```python
from build123d import *

# Parameters (mm, degrees)
SKETCH1_W               = 120.517011816
SKETCH1_H               = 193.423301163
BOSS_EXTRUDE1_DEPTH     = 75
SKETCH1_3_W             = 118.517011816
SKETCH1_3_H             = 191.423301163
CUT_EXTRUDE1_DEPTH      = 70
BOSS_EXTRUDE2_DEPTH     = 1
CUT_EXTRUDE4_DEPTH      = 137.495747048
CUT_EXTRUDE4_DEPTH_BACK = 137.495747048
CUT_EXTRUDE6_DEPTH      = 10
CUT_EXTRUDE3_DEPTH      = 10


with BuildPart() as part:
    # Sketch1 → Boss-Extrude1 (new body)
    with BuildSketch(Plane.XY):
        with Locations((0.026299542, -0.057021664)):
            Rectangle(SKETCH1_W, SKETCH1_H)
    extrude(amount=BOSS_EXTRUDE1_DEPTH)

    # Sketch1_3 → Cut-Extrude1 (cut)
    with BuildSketch(Plane.XY):
        with Locations((0.026299542, -0.057021664)):
            Rectangle(SKETCH1_3_W, SKETCH1_3_H)
    extrude(amount=CUT_EXTRUDE1_DEPTH, mode=Mode.SUBTRACT)

    # Sketch2 → Boss-Extrude2 (add)
    with BuildSketch(Plane(origin=(0, 96.654628917, 0), x_dir=(1, 0, 0), z_dir=(0, 1, 0))):
        with BuildLine():
            Line((-5.120692539, 0), (4.878786885, 0))
            ThreePointArc((4.878786885, 0), (-0.120952827, 5.051017752), (-5.120692539, 0))
        make_face()
    extrude(amount=-BOSS_EXTRUDE2_DEPTH)

    # Sketch4_2 → Cut-Extrude4 (cut, two sides: drawn at the far end of the back side and taken through both)
    with BuildSketch(Plane(origin=(0, 0, 70), x_dir=(-1, 0, 0), z_dir=(0, 0, -1)).offset(-CUT_EXTRUDE4_DEPTH_BACK)):
        with BuildLine():
            Line((-16.236705508, 8.803847843), (-16.236705508, 26.966349614))
            add(Edge.make_bspline(
                [(10.654600955, 26.966349614), (10.654600955, 37.042694246), (-2.791052277, 37.042694246), (-16.236705508, 37.042694246), (-16.236705508, 26.966349614)],
                knots=[3.141592654, 3.141592654, 3.141592654, 4.71238898, 4.71238898, 6.283185307, 6.283185307, 6.283185307], degree=2, weights=[1, 0.707106781, 1, 0.707106781, 1]))
            Line((10.654600955, 26.966349614), (10.654600955, 8.803847843))
            add(Edge.make_bspline(
                [(-16.236705508, 8.803847843), (-16.236705508, 0.726850718), (-2.791052277, 0.726850718), (10.654600955, 0.726850718), (10.654600955, 8.803847843)],
                knots=[0, 0, 0, 1.570796327, 1.570796327, 3.141592654, 3.141592654, 3.141592654], degree=2, weights=[1, 0.707106781, 1, 0.707106781, 1]))
        make_face()
    extrude(amount=CUT_EXTRUDE4_DEPTH + CUT_EXTRUDE4_DEPTH_BACK, mode=Mode.SUBTRACT)

    # Sketch6 → Cut-Extrude6 (cut, symmetric)
    with BuildSketch(Plane(origin=(0, 96.654628917, 0), x_dir=(1, 0, 0), z_dir=(0, 1, 0))):
        with BuildLine():
            add(Edge.make_bspline(
                [(14.607126744, -59.625274066), (14.607126744, -59.996423236), (14.655753616, -60.360654617), (14.797863596, -60.897161426), (14.856849596, -61.074344505), (14.9984446, -61.42534999), (15.081484622, -61.59993657), (15.36467279, -62.113067792), (15.595340891, -62.436179632), (16.002179988, -62.893279801), (16.148006268, -63.041018505), (16.460654262, -63.326982062), (16.627232407, -63.464794132), (17.147507806, -63.854923379), (17.524850755, -64.087300386), (18.13663611, -64.394273167), (18.349476527, -64.490080589), (18.784383, -64.664483705), (19.006061662, -64.743067855), (19.683439186, -64.953650763), (20.15136039, -65.060723061), (21.120984475, -65.205972716), (21.610951465, -65.242067863), (22.343801341, -65.24262469), (22.588258242, -65.23389357), (23.07752571, -65.198266478), (23.323602223, -65.171129385), (24.04825359, -65.063568363), (24.515989992, -64.95745801), (25.42125883, -64.677606952), (25.862082399, -64.501556566), (26.676946551, -64.094389908), (27.055163448, -63.862622522), (27.577987155, -63.47204045), (27.745226091, -63.334101772), (28.057458003, -63.04956749), (28.20337387, -62.902368403), (28.611107489, -62.446258784), (28.843853735, -62.121803074), (29.223293972, -61.437507678), (29.365303175, -61.086770508), (29.50923045, -60.548226995), (29.545607426, -60.366624344), (29.594557113, -59.999133521), (29.606945323, -59.813278674), (29.607483579, -59.261578321), (29.560066597, -58.897421315), (29.417460244, -58.356636708), (29.357535803, -58.176377178), (29.214631397, -57.822433786), (29.132057014, -57.649371871), (28.851902237, -57.14158682), (28.62220127, -56.818155033), (28.211284873, -56.35633663), (28.063808332, -56.207204664), (27.752933385, -55.923051914), (27.424862325, -55.651543664), (27.062811294, -55.405021279), (26.683482778, -55.171203227), (26.483999533, -55.060101063), (25.869660817, -54.752095839), (25.43867317, -54.579379415), (24.534710357, -54.297863736), (24.056862603, -54.188834821), (23.095878735, -54.045053542), (22.609683495, -54.008631963), (21.871731404, -54.007851656), (21.623217783, -54.016782482), (21.133474519, -54.052593794), (20.891228101, -54.079395605), (20.172200955, -54.185935333), (19.702248556, -54.291799913), (18.786992965, -54.574854931), (18.355286434, -54.747702842), (17.745137882, -55.052178339), (17.548036265, -55.161259722), (17.166702804, -55.394972905), (16.982301592, -55.51989473), (16.460673231, -55.909894482), (16.150371394, -56.192508636), (15.604234807, -56.802703679), (15.368452042, -57.132300307), (14.993164183, -57.809021831), (14.850249749, -58.159277139), (14.656312657, -58.884223774), (14.607126744, -59.254124896), (14.607126744, -59.625274066)],
                knots=[0, 0, 0, 0, 0.03125, 0.03125, 0.046875, 0.046875, 0.0625, 0.0625, 0.09375, 0.09375, 0.109375, 0.109375, 0.125, 0.125, 0.15625, 0.15625, 0.171875, 0.171875, 0.1875, 0.1875, 0.21875, 0.21875, 0.25, 0.25, 0.265625, 0.265625, 0.28125, 0.28125, 0.3125, 0.3125, 0.34375, 0.34375, 0.375, 0.375, 0.390625, 0.390625, 0.40625, 0.40625, 0.4375, 0.4375, 0.46875, 0.46875, 0.484375, 0.484375, 0.5, 0.5, 0.53125, 0.53125, 0.546875, 0.546875, 0.5625, 0.5625, 0.59375, 0.59375, 0.609375, 0.609375, 0.625, 0.640625, 0.640625, 0.65625, 0.65625, 0.6875, 0.6875, 0.71875, 0.71875, 0.75, 0.75, 0.765625, 0.765625, 0.78125, 0.78125, 0.8125, 0.8125, 0.84375, 0.84375, 0.859375, 0.859375, 0.875, 0.875, 0.90625, 0.90625, 0.9375, 0.9375, 0.96875, 0.96875, 1, 1, 1, 1], degree=3))
        make_face()
    extrude(amount=CUT_EXTRUDE6_DEPTH, both=True, mode=Mode.SUBTRACT)

    # Sketch4 → Cut-Extrude3 (cut, symmetric)
    with BuildSketch(Plane(origin=(0, 0, 70), x_dir=(-1, 0, 0), z_dir=(0, 0, -1))):
        with BuildLine():
            Line((-16.236705508, 8.803847843), (-16.236705508, 26.966349614))
            add(Edge.make_bspline(
                [(10.654600955, 26.966349614), (10.654600955, 37.042694246), (-2.791052277, 37.042694246), (-16.236705508, 37.042694246), (-16.236705508, 26.966349614)],
                knots=[3.141592654, 3.141592654, 3.141592654, 4.71238898, 4.71238898, 6.283185307, 6.283185307, 6.283185307], degree=2, weights=[1, 0.707106781, 1, 0.707106781, 1]))
            Line((10.654600955, 26.966349614), (10.654600955, 8.803847843))
            add(Edge.make_bspline(
                [(-16.236705508, 8.803847843), (-16.236705508, 0.726850718), (-2.791052277, 0.726850718), (10.654600955, 0.726850718), (10.654600955, 8.803847843)],
                knots=[0, 0, 0, 1.570796327, 1.570796327, 3.141592654, 3.141592654, 3.141592654], degree=2, weights=[1, 0.707106781, 1, 0.707106781, 1]))
        make_face()
    extrude(amount=CUT_EXTRUDE3_DEPTH, both=True, mode=Mode.SUBTRACT)


solid = part.part
```
Work out the finished part from the listing and answer in its coordinate system (mm). A direction names the side the tool comes from. Round coordinates to 2 decimals unless told otherwise and drop trailing zeros. Write each loop counter-clockwise with the first axis right and the second up, starting at its lowest first coordinate (ties: lowest second). Pieces come first, ordered by that corner, then holes.
1) A flat-ended cylindrical pin translates along its axis: P1, Ø12, axis at x = 44, y = -22.5, coming from the -Z side. Find the tip coordinate at first contact, or state that the pin passes through.
2) A cutting plane is placed at B-B on z = 14. Determine the outline of the cut face in (x, y), and give its area (3 significant figures).
3) A cutting plane is placed at D-D on x = 38. Determine the outline of the cut face in (y, z).
4) A cutting plane is placed at A-A on y = 14.5. Determine the outline of the cut face in (x, z), and give its area (3 significant figures).
5) Consider probe 1 along X at (y, z) = (22, 56.5); probe 2 along Y at (x, z) = (-45.5, 7.5); probe 3 along Z at (x, y) = (37.5, -83.5). Determine where each line is inside the solid, lowest interval first.
6) Determine the mould class of faces 4 (the face through (-0.01, 96.16, -5.05)), 5 (the face through (-60.232, -1, 37)), 6 (the face through (-59.232, -1, 35)) for opening direction X: pulls with the +X half, pulls with the -X half, needs draft (parallel to the pull), parting line crosses it, or undercut.
7) Which of the six approach directions +Z, -Z, +X, -X, +Y, -Y give full straight-line access (tool end or side, diameter ignored) to faces 1 (the face through (-1, -95.769, 35)), 2 (the face through (-14, 1, 75)), 3 (the face through (-10.655, 18, 73))?
8) A cutting plane is placed at C-C on y = -43. Determine the outline of the cut face in (x, z).
Entries:
1. P1: stops at z = 70
2. outline: (-60.23, -96.77) - (60.28, -96.77) - (60.28, 96.65) - (-60.23, 96.65) - close; hole (-59.23, -95.77) - (59.28, -95.77) - (59.28, 95.65) - (-59.23, 95.65) - close
2. area: 624 mm2
3. outline: (-96.77, 0) - (-95.77, 0) - (-95.77, 70) - (95.65, 70) - (95.65, 0) - (96.65, 0) - (96.65, 75) - (-96.77, 75) - close
4. outline: (-60.23, 0) - (-59.23, 0) - (-59.23, 70) - (-10.65, 70) - (-10.65, 75) - (-60.23, 75) - close; (16.24, 70) - (59.28, 70) - (59.28, 0) - (60.28, 0) - (60.28, 75) - (16.24, 75) - close
4. area: 608 mm2
5. probe 1: x = -60.23 to -59.23, 59.28 to 60.28
5. probe 2: y = -96.77 to -95.77, 95.65 to 96.65
5. probe 3: z = 70 to 75
6. face 4: parting line crosses it
6. face 5: pulls with the -X half
6. face 6: undercut
7. face 1: -Z
7. face 2: +Z, +X, -X, +Y, -Y
7. face 3: +Z, -Z
8. outline: (-60.23, 0) - (-59.23, 0) - (-59.23, 70) - (59.28, 70) - (59.28, 0) - (60.28, 0) - (60.28, 75) - (-60.23, 75) - close
